Verification items for the finished model (mm, model axes). A direction names the side the tool comes from. Round coordinates to 2 decimals unless told otherwise and drop trailing zeros. Write each loop counter-clockwise with the first axis right and the second up, starting at its lowest first coordinate (ties: lowest second). Pieces come first, ordered by that corner, then holes. Notation, with made-up numbers: M 75.5,36.5 L 111.5,36.5 A11 cw 111.5,48.5 Z; hole C 89.25,20.25 d2. An arc over 180 degrees is marked long. One line per question, with ' | ' between items. Start each with the question number.
Q1. Thickness scan on line 1 along Y through (x, z) = (0.9, 0); line 2 along Y through (x, z) = (1.25, 14); line 3 along Z through (x, y) = (0.25, 19.5). Record the ranges inside material, lowest first. Write a range as from..to.
Q2. Gauge pin test, flat ends, axial feed: pin 1 (5 mm diameter, centred on y = -10.38, z = 0, fed in from +X); pin 2 (3 mm diameter, centred on y = 12.5, z = -14.5, fed in from -X); pin 3 (0.9 mm diameter, centred on x = 1.5, z = 21.5, fed in from +Y). Record the tip position at first contact, or that the pin passes through.
Q3. Cross-section at D-D (y = 0.5). Record the boundary of the cut face in (x, z), then the cut area to 3 significant figures.
Q4. Cross-section at B-B (z = 14). Record the boundary of the cut face in (x, y).
Q5. Cross-section at C-C (x = 1.4). Record the boundary of the cut face in (y, z).
Q6. Tool access check on faces 1 (the face through (2, 18, -24.5)), 2 (the face through (1, -10.382, -18)), 3 (the face through (1.479, 45.616, -0.132)), 4 (the face through (1, -10.382, 18)), 5 (the face through (1, 39.618, 18)). Record the directions out of +Z, -Z, +X, -X, +Y, -Y that give a thin tool (end or side, any length) a straight path to the whole face; none if there is none.
Q7. Cross-section at A-A (y = 19). Record the boundary of the cut face in (x, z), then the cut area to 3 significant figures.
Q8. Release check for a two-part mould opening along Z. For faces 6 (the face through (1, 39.618, -18)), 7 (the face through (1, 15, 35)), 8 (the face through (2, 17, -11.5)) record: released by +Z, released by -Z, zero draft, split by the parting line, or undercut.
from build123d import *

# Parameters (mm, degrees)
BOSS_EXTRUDE1_DEPTH = 3
SKETCH2_R           = 1.5
SKETCH2_R_2         = 10.5
CUT_EXTRUDE1_DEPTH  = 4


with BuildPart() as part:
    # Sketch1 → Boss-Extrude1 (new body)
    with BuildSketch(Plane(origin=(0, 0, 0), x_dir=(0, 0, -1), z_dir=(1, 0, 0))):
        with BuildLine():
            Line((35, -5.382304056), (35, 34.617695944))
            ThreePointArc((35, 34.617695944), (33.535533906, 38.15322985), (30, 39.617695944))
            Line((30, 39.617695944), (6, 39.617695944))
            ThreePointArc((6, 39.617695944), (0, 45.617695944), (-6, 39.617695944))
            Line((-6, 39.617695944), (-30, 39.617695944))
            ThreePointArc((-30, 39.617695944), (-33.535533906, 38.15322985), (-35, 34.617695944))
            Line((-35, 34.617695944), (-35, -5.382304056))
            ThreePointArc((-35, -5.382304056), (-33.535533906, -8.917837962), (-30, -10.382304056))
            Line((-30, -10.382304056), (-6, -10.382304056))
            ThreePointArc((-6, -10.382304056), (0, -16.382304056), (6, -10.382304056))
            Line((6, -10.382304056), (30, -10.382304056))
            ThreePointArc((30, -10.382304056), (33.535533906, -8.917837962), (35, -5.382304056))
        make_face()
    extrude(amount=BOSS_EXTRUDE1_DEPTH)

    # Sketch2 → Cut-Extrude1 (cut, through all)
    with BuildSketch(Plane(origin=(3, 0, 0), x_dir=(0, 0, -1), z_dir=(1, 0, 0))):
        with Locations((0, 39.617695944)):
            Circle(SKETCH2_R)
        with Locations((0, -10.382304056)):
            Circle(SKETCH2_R)
        with Locations((-14, 19)):
            Circle(SKETCH2_R_2)
        with BuildLine():
            Line((11.5, 30), (24.5, 30))
            Line((24.5, 30), (24.5, 5))
            ThreePointArc((24.5, 5), (18, -1.5), (11.5, 5))
            Line((11.5, 5), (11.5, 30))
        make_face()
    extrude(amount=-CUT_EXTRUDE1_DEPTH, mode=Mode.SUBTRACT)


solid = part.part
Determined:
1) line 1: y = -16.38..-11.88, -8.88..38.12, 41.12..45.62 | line 2: y = -10.38..8.5, 29.5..39.62 | line 3: z = -35..-24.5, -11.5..3.51, 24.49..35
2) pin 1: stops at x = 3 | pin 2: passes through | pin 3: stops at y = 39.62
3) outline: M 0,-35 L 3,-35 L 3,-22.69 L 0,-22.69 Z; M 0,-13.31 L 3,-13.31 L 3,35 L 0,35 Z | area: 182 mm²
4) outline: M 0,-10.38 L 3,-10.38 L 3,8.5 L 0,8.5 Z; M 0,29.5 L 3,29.5 L 3,39.62 L 0,39.62 Z
5) outline: M -10.38,-30 A5 ccw -5.38,-35 L 34.62,-35 A5 ccw 39.62,-30 L 39.62,-6 A6 ccw 39.62,6 L 39.62,30 A5 ccw 34.62,35 L -5.38,35 A5 ccw -10.38,30 L -10.38,6 A6 ccw -10.38,-6 Z; hole C -10.38,0 d3; hole M 5,-24.5 L 30,-24.5 L 30,-11.5 L 5,-11.5 A6.5 ccw Z; hole C 19,14 d21; hole C 39.62,0 d3
6) face 1: +X, -X | face 2: -Z, +X, -X, -Y | face 3: +X, -X, +Y | face 4: +Z, +X, -X, -Y | face 5: +Z, +X, -X, +Y
7) outline: M 0,-35 L 3,-35 L 3,-24.5 L 0,-24.5 Z; M 0,-11.5 L 3,-11.5 L 3,3.5 L 0,3.5 Z; M 0,24.5 L 3,24.5 L 3,35 L 0,35 Z | area: 108 mm²
8) face 6: zero draft | face 7: released by +Z | face 8: undercut
